```python
from build123d import *

# Parameters (mm, degrees)
F0_W     = 15
F0_H     = 3.81
F1_DEPTH = 3.81


# Not quite as in the source:
# - a feature names something its author has since deleted; it is built from what else it names


with BuildPart() as f1:
    # F0 (on Top) → F1 (new body)
    with BuildSketch(Plane.XY):
        with Locations((-45, -27.905)):
            Rectangle(F0_W, F0_H)
        Polygon((-37.5, -26), (62.5, -26), (61.059539805, -20.23815922), (57.4215054295, -5.6860217178), (54.9434199682, 4.226320127), (51.3053855927, 18.7784576292), (49.5, 26), (-24.5351687992, 26), (-39.5349438522, 26), (-49.5349438522, 26), (-62.5, -26), (-52.5, -26), align=None)
        Polygon((61.059539805, -20.23815922), (62.5, -19.8780441712), (62.5, -10.2909675664), (61.117748355, -4.7619609864), (57.4215054295, -5.6860217178), align=None)
        Polygon((51.3053855927, 18.7784576292), (54.9434199682, 4.226320127), (58.6396628938, 5.1503808584), (55.0016285183, 19.7025183606), align=None)
        Polygon((62.5, -10.2909675664), (62.5, -19.8780441712), (64.7557827306, -19.3140984886), align=None)
        Polygon((-39.5349438522, 29.81), (-39.5349438522, 26), (-24.5351687992, 26), (-24.5351687992, 29.7278515898), align=None)
    extrude(amount=F1_DEPTH)


solid = f1.part
```
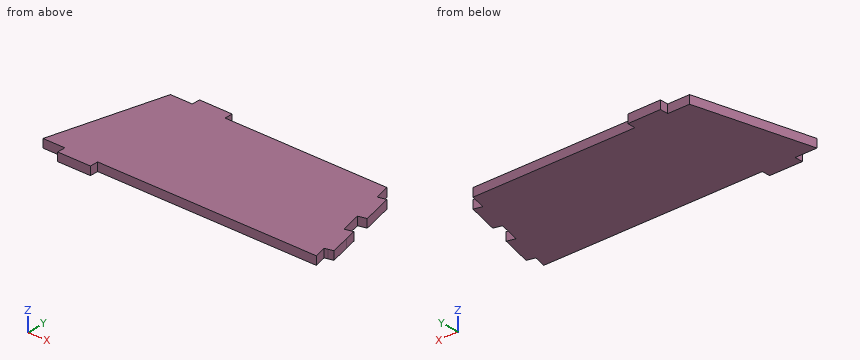
Geometry: final body of the model. Coordinates: model frame, mm. Round coordinates to 2 decimals unless told otherwise and drop trailing zeros. Order: outer loops, then holes, each group sorted by start corner. A loop starts at its lowest first (then second) coordinate and runs counter-clockwise, first axis right, second up. Notation, with made-up numbers: (56.25, 43) -> (89.25, 43) arc R19 cw to (89.25, 79) -> close; hole circle Ø3 at (-2, 26.5). An arc over 180 degrees is marked (long way). Use one line per item in the form item = value.
(1) Ray query, probe 1 along Y at (x, z) = (46.5, 2); probe 2 along Y at (x, z) = (-48, 1.5); probe 3 along X at (y, z) = (14, 2.95). Return the intervals inside material, ascending. Write a range as [from, to].
Results list:
probe_1 = [-26, 26]
probe_2 = [-29.81, 26]
probe_3 = [-52.53, 56.43]
(2) Section C-C on y = -17.5. Return loops of the section in (x, z), and give its area (3 significant figures).
Results list:
outline = (-60.38, 0) -> (64.3, 0) -> (64.3, 3.81) -> (-60.38, 3.81) -> close
area = 475 mm^2
(3) Section B-B on x = 43.5. Return loops of the section in (y, z).
Results list:
outline = (-26, 0) -> (26, 0) -> (26, 3.81) -> (-26, 3.81) -> close
(4) First-contact query: pin 1 Ø1.9 at (y, z) = (28, 2) entering from +X; pin 2 Ø1.1 at (y, z) = (-27.5, 1.5) entering from +X; pin 3 Ø1.1 at (y, z) = (-27.5, 2) entering from -X. Flat tips, straight axial feed; report the tip coordinate or a pass-through.
Results list:
pin_1 = -24.54
pin_2 = -37.5
pin_3 = -52.5
(5) Section A-A on z = 1.9. Return loops of the section in (x, y).
Results list:
outline = (-62.5, -26) -> (-52.5, -26) -> (-52.5, -29.81) -> (-37.5, -29.81) -> (-37.5, -26) -> (62.5, -26) -> (61.06, -20.24) -> (64.76, -19.31) -> (61.12, -4.76) -> (57.42, -5.69) -> (54.94, 4.23) -> (58.64, 5.15) -> (55, 19.7) -> (51.31, 18.78) -> (49.5, 26) -> (-24.54, 26) -> (-24.54, 29.73) -> (-39.53, 29.81) -> (-39.53, 26) -> (-49.53, 26) -> close
